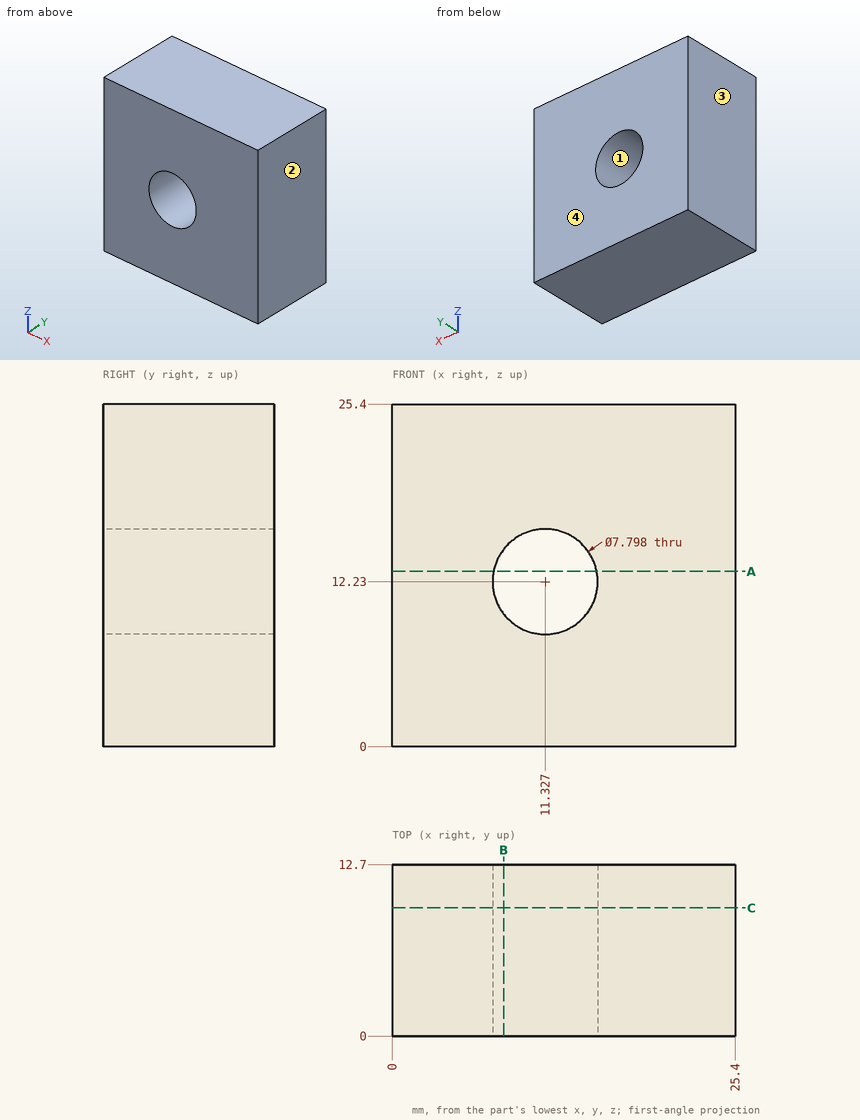
For this review, use the dimensioned drawing (mm, ordinates from the lowest corner) and the shaded views. Round coordinates to 2 decimals unless told otherwise and drop trailing zeros. Order: outer loops, then holes, each group sorted by start corner. A loop starts at its lowest first (then second) coordinate and runs counter-clockwise, first axis right, second up. Notation, with made-up numbers: (-27.75, 37) -> (-12.75, 37) arc R18 ccw to (-12.75, 64) -> close; hole circle Ø10 at (26, 29). An arc over 180 degrees is marked (long way). Write item = value, one per line. Start each with the question number.
Item 1: Consider section C-C on y = 9.5. Write out the cut boundary in (x, z).
Item 2: Consider section B-B on x = 8.25. Write out the cut boundary in (y, z) (1 decimal).
Item 3: Mouldability with a two-part tool opening along X and no side actions: class the marked faces 1, 2, 3 and 4 as released by +X, released by -X, zero draft, split by the parting line, or undercut.
Item 4: For line 1 along X through (y, z) = (12, 12.25); line 2 along Z through (x, y) = (11.25, 8.75); line 3 along X through (y, z) = (3.5, 13.75), list the stretches that pass through material, from the lowest coordinate up.
Item 5: Consider section A-A on z = 13. Write out the cut boundary in (x, y) (1 decimal).
Item 6: Clearance check with a flat-ended pin moving along its axis: pin 1 Ø4.5 at (x, z) = (11.33, 12.23) entering from +Y. State where the tip first meets the part, or that it passes through.
Conclusion:
q1.outline = (0, 0) -> (25.4, 0) -> (25.4, 25.4) -> (0, 25.4) -> close; hole circle Ø7.8 at (11.33, 12.23)
q2.outline = (0, 0) -> (12.7, 0) -> (12.7, 9.8) -> (0, 9.8) -> close; (0, 14.6) -> (12.7, 14.6) -> (12.7, 25.4) -> (0, 25.4) -> close
q3.face_1 = undercut
q3.face_2 = released by +X
q3.face_3 = released by -X
q3.face_4 = zero draft
q4.line_1 = 0 to 7.43, 15.23 to 25.4
q4.line_2 = 0 to 8.33, 16.13 to 25.4
q4.line_3 = 0 to 7.74, 14.92 to 25.4
q5.outline = (0, 0) -> (7.5, 0) -> (7.5, 12.7) -> (0, 12.7) -> close; (15.1, 0) -> (25.4, 0) -> (25.4, 12.7) -> (15.1, 12.7) -> close
q6.pin_1 = through
